Answer from the drawing. Dimensions are ordinates in mm from the lowest x, y and z of the part. A direction names the side the tool comes from. Give positions to 0.01 mm unless a question says otherwise; leave off trailing zeros. Order: outer loops, then holes, each group sorted by start corner. A loop starts at its lowest first (then second) coordinate and runs counter-clockwise, first axis right, second up. Notation, with made-up numbers: (2, -38) - (34, -38) arc R20 cw to (34, -27) - close; hole circle Ø11 at (-9.75, 34). An arc over 180 degrees is marked (long way). Answer in a Markdown table with one row per item.
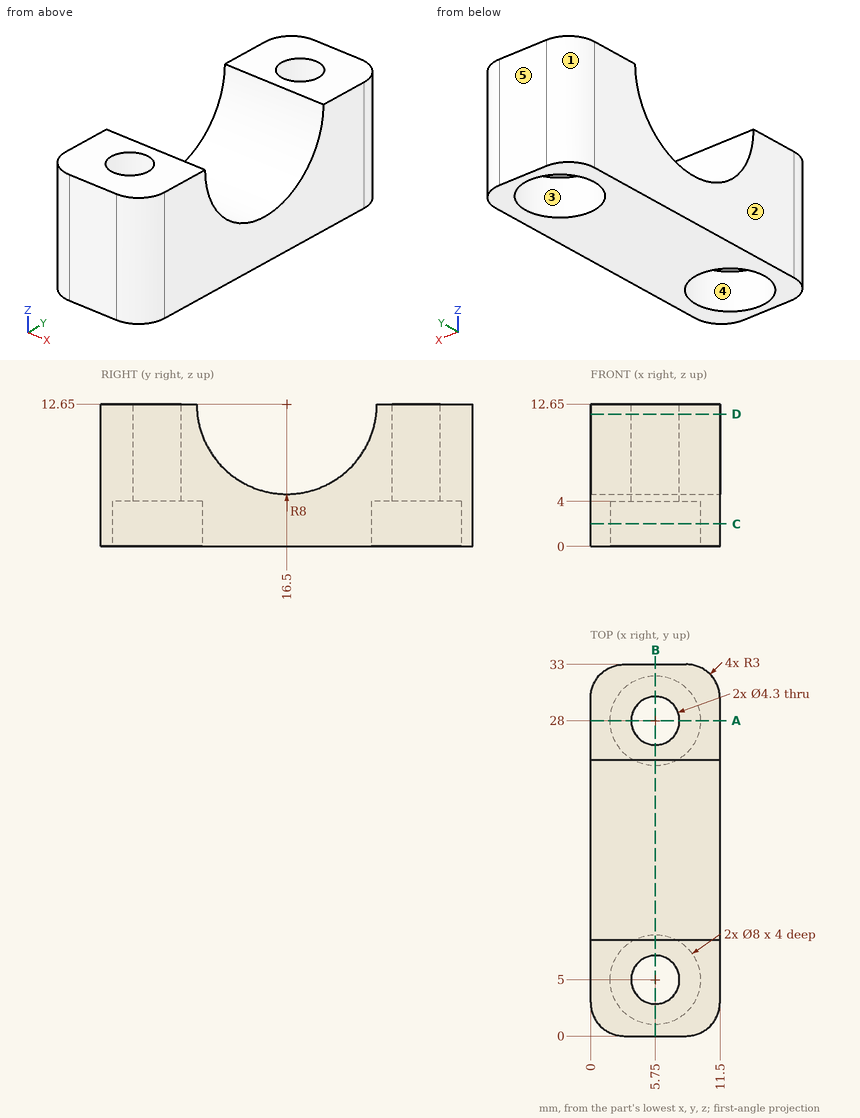
Item 1: Determine the mould class of the marked faces 1, 2 and 3 for opening direction Y: pulls with the +Y half, pulls with the -Y half, needs draft (parallel to the pull), parting line crosses it, or undercut.
Answer block:
| item | result |
|---|---|
| face 1 | pulls with the +Y half |
| face 2 | needs draft |
| face 3 | undercut |
Item 2: Find section A-A on y = 28. Write down the section's boundary in (x, z), then the cut area to 3 significant figures.
Answer block:
| item | result |
|---|---|
| outline | (0, 0) - (1.75, 0) - (1.75, 4) - (3.6, 4) - (3.6, 12.65) - (0, 12.65) - close; (7.9, 4) - (9.75, 4) - (9.75, 0) - (11.5, 0) - (11.5, 12.65) - (7.9, 12.65) - close |
| area | 76.3 mm² |
Item 3: Find section D-D on z = 11.75. Write down the section's boundary in (x, y).
Answer block:
| item | result |
|---|---|
| outline | (0, 3) arc R3 ccw to (3, 0) - (8.5, 0) arc R3 ccw to (11.5, 3) - (11.5, 8.55) - (0, 8.55) - close; (0, 24.45) - (11.5, 24.45) - (11.5, 30) arc R3 ccw to (8.5, 33) - (3, 33) arc R3 ccw to (0, 30) - close; hole circle Ø4.3 at (5.75, 5); hole circle Ø4.3 at (5.75, 28) |
Item 4: Find section B-B on x = 5.75. Write down the section's boundary in (y, z).
Answer block:
| item | result |
|---|---|
| outline | (0, 0) - (1, 0) - (1, 4) - (2.85, 4) - (2.85, 12.65) - (0, 12.65) - close; (7.15, 4) - (9, 4) - (9, 0) - (24, 0) - (24, 4) - (25.85, 4) - (25.85, 12.65) - (24.5, 12.65) arc R8 cw to (8.5, 12.65) - (7.15, 12.65) - close; (30.15, 4) - (32, 4) - (32, 0) - (33, 0) - (33, 12.65) - (30.15, 12.65) - close |
Item 5: Each of these flat-tipped pins is pushed along its axis until it touches: P1, Ø1, axis at x = 10, z = 5, coming from the +Y side; P2, Ø1, axis at y = 16, z = 6.5, coming from the -X side; P3, Ø2.5, axis at x = 7, y = 5, coming from the -Z side. Where does it stop, or does it pass through?
Answer block:
| item | result |
|---|---|
| P1 | y = 32.83 |
| P2 | through |
| P3 | z = 4 |
Item 6: Consider line 1 (Y direction, x = 5.75, z = 3.2); line 2 (Y direction, x = 2.5, z = 2.5); line 3 (Y direction, x = 5.75, z = 7.5). Determine where each line is inside the solid, lowest interval first.
Answer block:
| item | result |
|---|---|
| line 1 | 0 to 1, 9 to 24, 32 to 33 |
| line 2 | 0.04 to 2.67, 7.33 to 25.67, 30.33 to 32.96 |
| line 3 | 0 to 2.85, 7.15 to 10.38, 22.62 to 25.85, 30.15 to 33 |
Item 7: Which of the six approach directions +Z, -Z, +X, -X, +Y, -Y give full straight-line access (tool end or side, diameter ignored) to the marked faces 4 and 5?
Answer block:
| item | result |
|---|---|
| face 4 | -Z |
| face 5 | +Z, -Z, +X, -X, +Y |
Item 8: Find section C-C on z = 2. Write down the section's boundary in (x, y).
Answer block:
| item | result |
|---|---|
| outline | (0, 3) arc R3 ccw to (3, 0) - (8.5, 0) arc R3 ccw to (11.5, 3) - (11.5, 30) arc R3 ccw to (8.5, 33) - (3, 33) arc R3 ccw to (0, 30) - close; hole circle Ø8 at (5.75, 5); hole circle Ø8 at (5.75, 28) |
